Design review of the part built by this model. Coordinates are the model's own, in mm. Give positions to 0.01 mm unless a question says otherwise; leave off trailing zeros. Write each loop counter-clockwise with the first axis right and the second up, starting at its lowest first coordinate (ties: lowest second). Pieces come first, ordered by that corner, then holes.
```python
from build123d import *

# Parameters (mm, degrees)
F0_R     = 2.65
F1_DEPTH = 18
F2_R     = 3.5
F3_DEPTH = 3
F4_R     = 3.5
F5_DEPTH = 3
F6_W     = 8
F6_H     = 7
F7_DEPTH = 3
F8_W     = 8
F8_H     = 7
F9_DEPTH = 3


with BuildPart() as f1:
    # F0 (on Top) → F1 (new body)
    with BuildSketch(Plane.XY):
        Circle(F0_R)
    extrude(amount=-F1_DEPTH)

    # F2 (on face) → F3 (join)
    with BuildSketch(Plane.XY):
        Circle(F2_R)
    extrude(amount=F3_DEPTH)

    # F4 (on face) → F5 (join)
    with BuildSketch(Plane(origin=(0, 0, -18), x_dir=(1, 0, 0), z_dir=(0, 0, -1))):
        Circle(F4_R)
    extrude(amount=F5_DEPTH)

    # F6 (on face) → F7 (join)
    with BuildSketch(Plane(origin=(0, 0, -21), x_dir=(1, 0, 0), z_dir=(0, 0, -1))):
        with Locations((4, 0)):
            Rectangle(F6_W, F6_H)
    extrude(amount=-F7_DEPTH)

    # F8 (on face) → F9 (join)
    with BuildSketch(Plane.XY.offset(3)):
        with Locations((4, 0)):
            Rectangle(F8_W, F8_H)
    extrude(amount=-F9_DEPTH)


solid = f1.part
```
(1) Consider section C-C, the plane z = -15.25. Give the boundary of the cut face in (x, y).
Resolved:
outline: circle Ø5.3 at (0, 0)
(2) Consider section A-A, the plane x = 6.25. Give the boundary of the cut face in (y, z), then the cut area to 3 significant figures.
Resolved:
outline: (-3.5, -21) - (3.5, -21) - (3.5, -18) - (-3.5, -18) - close; (-3.5, 0) - (3.5, 0) - (3.5, 3) - (-3.5, 3) - close
area: 42.0 mm2
(3) To check wall thickness, follow L1, parallel to Z at x = 7.5, y = 2.25; L2, parallel to X at y = -1, z = -1; L3, parallel to X at y = -0.25, z = -5.5. State the ranges of each line that lie inside material, in increasing order.
Resolved:
L1: z = -21 to -18, 0 to 3
L2: x = -2.45 to 2.45
L3: x = -2.64 to 2.64
(4) Mouldability with a two-part tool opening along Z and no side actions: class faces 1 (the face through (4, -3.5, -20)), 2 (the face through (2, 0, 3)), 3 (the face through (2.45, -1.01, -8.87)), 4 (the face through (3, 0, 0)) as pulls with the +Z half, pulls with the -Z half, needs draft (parallel to the pull), parting line crosses it, or undercut.
Resolved:
face 1: needs draft
face 2: pulls with the +Z half
face 3: undercut
face 4: undercut
(5) Consider section D-D, the plane x = 0.5. Give the boundary of the cut face in (y, z), then the cut area to 3 significant figures.
Resolved:
outline: (-3.5, -21) - (3.5, -21) - (3.5, -18) - (2.6, -18) - (2.6, 0) - (3.5, 0) - (3.5, 3) - (-3.5, 3) - (-3.5, 0) - (-2.6, 0) - (-2.6, -18) - (-3.5, -18) - close
area: 136 mm2
(6) Clearance check with flat-ended pins moving along their axes: P1, Ø3, axis at y = -2.5, z = -0.5, coming from the -X side; P2, Ø2, axis at x = 3, z = -6.5, coming from the +Y side; P3, Ø2, axis at x = 2, z = -7.5, coming from the -Y side. State where each tip first meets the part, or that it passes through.
Resolved:
P1: stops at x = -3.33
P2: stops at y = 1.74
P3: stops at y = -2.45
(7) Consider section B-B, the plane y = 0. Give the boundary of the cut face in (x, z).
Resolved:
outline: (-3.5, -21) - (8, -21) - (8, -18) - (2.65, -18) - (2.65, 0) - (8, 0) - (8, 3) - (-3.5, 3) - (-3.5, 0) - (-2.65, 0) - (-2.65, -18) - (-3.5, -18) - close
